Job drawing, mm, ordinate dimensions from the low corner. One solid piece. Give positions to 0.01 mm unless a question says otherwise; leave off trailing zeros. Write each loop counter-clockwise with the first axis right and the second up, starting at its lowest first coordinate (ties: lowest second). Pieces come first, ordered by that corner, then holes. Notation, with made-up numbers: M 61,5 L 108,5 A19 ccw 108,19 Z; hole C 24,29 d5. An arc over 180 degrees is marked long. Answer as CSV lines item,"result". Start each with the question number.
1) Slice it at C-C, the plane y = 4.1. Give the cut face in (x, z).
2) Wall check: line 1 along Z through (x, y) = (25.5, 4.5); line 2 along X through (y, z) = (5.1, 15.5); line 3 along Y through (x, z) = (17, 11.5). Give the ranges that are in metal, low to high. Write a range as from..to.
3) Mould opens along Z. For the marked faces 1 and 2 say: pulls with the +Z half, pulls with the -Z half, needs draft (parallel to the pull), parting line crosses it, or undercut.
4) Pin check, flat tips, straight feed: pin 1 Ø1.8 at (x, y) = (13.5, 1) entering from +Z; pin 2 Ø12 at (x, z) = (23, 19.5) entering from -Y. Stop position of each tip, or through.
5) Slice it at A-A, the plane z = 17. Give the cut face in (x, y).
6) Slice it at D-D, the plane x = 15. Give the cut face in (y, z).
7) Slice it at B-B, the plane x = 7.5. Give the cut face in (y, z).
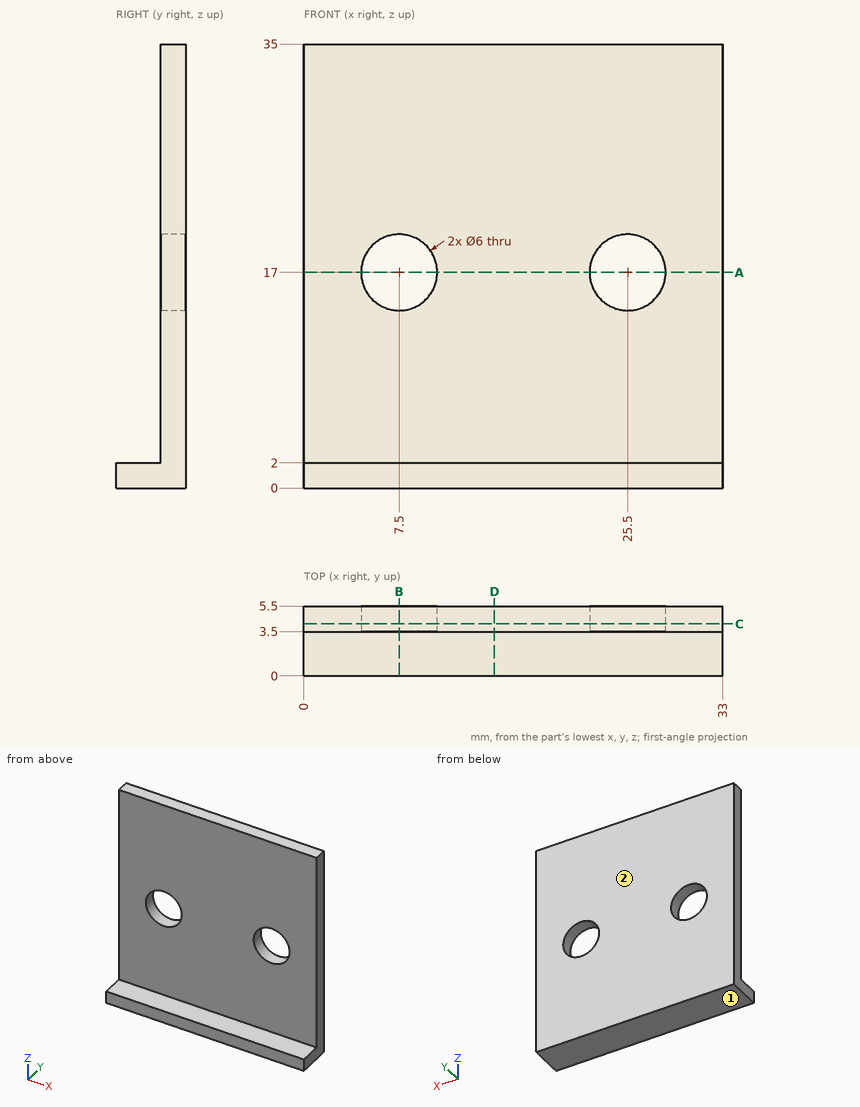
Found:
1,outline,"M 0,0 L 33,0 L 33,35 L 0,35 Z; hole C 7.5,17 d6; hole C 25.5,17 d6"
2,line 1,"0..14, 20..35"
2,line 2,"0..4.9, 10.1..22.9, 28.1..33"
2,line 3,"3.5..5.5"
3,face 1,"pulls with the -Z half"
3,face 2,"needs draft"
4,pin 1,"z = 2"
4,pin 2,"y = 3.5"
5,outline,"M 0,3.5 L 4.5,3.5 L 4.5,5.5 L 0,5.5 Z; M 10.5,3.5 L 22.5,3.5 L 22.5,5.5 L 10.5,5.5 Z; M 28.5,3.5 L 33,3.5 L 33,5.5 L 28.5,5.5 Z"
6,outline,"M 0,0 L 5.5,0 L 5.5,35 L 3.5,35 L 3.5,2 L 0,2 Z"
7,outline,"M 0,0 L 5.5,0 L 5.5,14 L 3.5,14 L 3.5,2 L 0,2 Z; M 3.5,20 L 5.5,20 L 5.5,35 L 3.5,35 Z"
